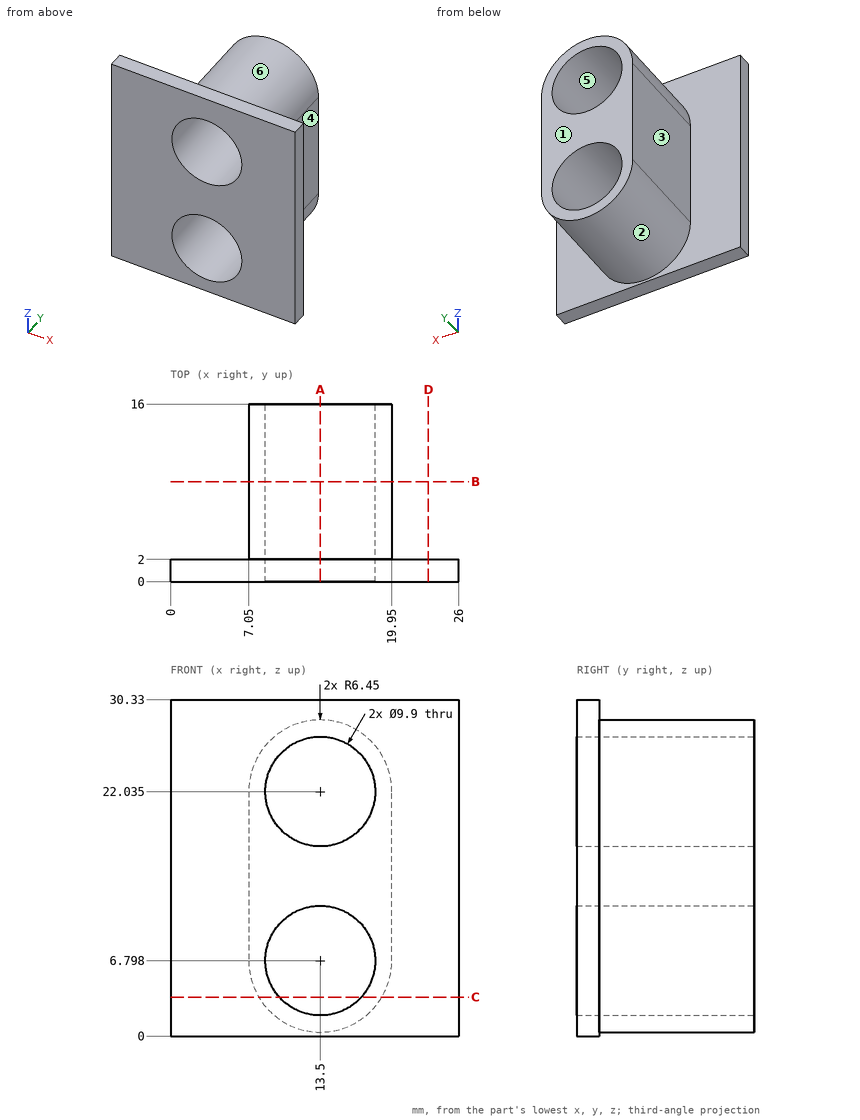
Answer from the drawing. Dimensions are ordinates in mm from the lowest x, y and z of the part. A direction names the side the tool comes from. Round coordinates to 2 decimals unless told otherwise and drop trailing zeros. Order: outer loops, then holes, each group sorted by start corner. A loop starts at its lowest first (then second) coordinate and runs counter-clockwise, first axis right, second up.
1) The part is cut by section C-C on z = 3.5. Write down the section's boundary in (x, y).
2) The part is cut by section A-A on x = 13.5. Write down the section's boundary in (y, z) (3 decimals).
3) Straight lines are drawn through the part: L1, parallel to Z at x = 13, y = 11.25; L2, parallel to Z at x = 9.5, y = 4.25 (3 decimals); L3, parallel to Y at x = 20.5, z = 14. For each, find the intervals that lie inside material, in ascending order.
4) The part is cut by section D-D on x = 23.25. Write down the section's boundary in (y, z), plus the area to 3 significant figures.
5) The part is cut by section B-B on y = 9. Write down the section's boundary in (x, z) (3 decimals), plus the area to 3 significant figures.
6) The mould has two halves that part along X. Classify the marked faces 4, 5 and 6: released by +X, released by -X, zero draft, split by the parting line, or undercut.
7) For the marked faces 1, 2 and 3, determine the directions among +Z, -Z, +X, -X, +Y, -Y from which every point of the face is accessible in a straight line to the end or side of a thin tool.
8) Flat-ended cylindrical pins translate along their axes: pin 1 (5 mm diameter, centred on x = 8, z = 23.5, fed in from -Y); pin 2 (4 mm diameter, centred on x = 17, y = 7.5, fed in from -Z); pin 3 (4 mm diameter, centred on x = 19.5, y = 13, fed in from -Z); pin 4 (4 mm diameter, centred on y = 7.5, z = 17.5, fed in from -X). Find the tip coordinate at first contact, or state that the pin passes through.
Resolved:
1. outline: (0, 0) - (9.81, 0) - (9.81, 16) - (7.96, 16) - (7.96, 2) - (0, 2) - close; (17.19, 0) - (26, 0) - (26, 2) - (19.04, 2) - (19.04, 16) - (17.19, 16) - close
2. outline: (0, 0) - (2, 0) - (2, 0.348) - (16, 0.348) - (16, 1.848) - (0, 1.848) - close; (0, 11.748) - (16, 11.748) - (16, 17.085) - (0, 17.085) - close; (0, 26.985) - (16, 26.985) - (16, 28.485) - (2, 28.485) - (2, 30.33) - (0, 30.33) - close
3. L1: z = 0.37 to 1.87, 11.72 to 17.11, 26.96 to 28.47
3. L2: z = 1.738 to 3.882, 9.714 to 19.119, 24.951 to 27.095
3. L3: y = 0 to 2
4. outline: (0, 0) - (2, 0) - (2, 30.33) - (0, 30.33) - close
4. area: 60.7 mm2
5. outline: (7.05, 6.798) arc R6.45 ccw to (19.95, 6.798) - (19.95, 22.035) arc R6.45 ccw to (7.05, 22.035) - close; hole circle Ø9.9 at (13.5, 6.798); hole circle Ø9.9 at (13.5, 22.035)
5. area: 173 mm2
6. face 4: released by +X
6. face 5: undercut
6. face 6: split by the parting line
7. face 1: +Z, -Z, +X, -X, +Y
7. face 2: -Z, +Y
7. face 3: +Z, -Z, -X, +Y
8. pin 1: stops at y = 0
8. pin 2: stops at z = 0.52
8. pin 3: stops at z = 1.74
8. pin 4: stops at x = 7.05
